```python
from build123d import *

# Parameters (mm, degrees)
SKETCH_1_W          = 120
SKETCH_1_H          = 40
EXTRUDE_1_DEPTH     = 25
SKETCH_2_R          = 2.75
CUT_EXTRUDE_1_DEPTH = 25
SKETCH_5_W          = 157.5
SKETCH_5_H          = 80
EXTRUDE_2_DEPTH     = 5
SKETCH_6_W          = 60
SKETCH_6_H          = 40
CUT_EXTRUDE_3_DEPTH = 20
FILLET_1_R          = 4
CHAMFER_1_SIZE      = 0.5


with BuildPart() as part:
    # 草图1 → 凸台-拉伸1 (new body)
    with BuildSketch(Plane(origin=(0, 0, 0), x_dir=(1, 0, 0), z_dir=(0, 1, 0))):
        Rectangle(SKETCH_1_W, SKETCH_1_H)
    extrude(amount=EXTRUDE_1_DEPTH)

    # 草图2 → 切除-拉伸1 (cut)
    with BuildSketch(Plane.XZ):
        with Locations(Location((-52.5, 11.75, 0), (0, 0, 270))):
            Circle(SKETCH_2_R)
        with Locations(Location((-52.5, -11.75, 0), (0, 0, 270))):
            Circle(SKETCH_2_R)
        with Locations(Location((52.5, -11.75, 0), (0, 0, 270))):
            Circle(SKETCH_2_R)
        with Locations(Location((52.5, 11.75, 0), (0, 0, 270))):
            Circle(SKETCH_2_R)
    extrude(amount=-CUT_EXTRUDE_1_DEPTH, mode=Mode.SUBTRACT)

    # 草图5 → 凸台-拉伸2 (add)
    with BuildSketch(Plane(origin=(0, 25, 0), x_dir=(1, 0, 0), z_dir=(0, 1, 0))):
        with Locations((0, 20)):
            Rectangle(SKETCH_5_W, SKETCH_5_H)
    extrude(amount=EXTRUDE_2_DEPTH)

    # 草图6 → 切除-拉伸3 (cut)
    with BuildSketch(Plane.XZ):
        Rectangle(SKETCH_6_W, SKETCH_6_H)
    extrude(amount=-CUT_EXTRUDE_3_DEPTH, mode=Mode.SUBTRACT)

    # 圆角1
    fillet_1_edges = [part.edges().sort_by_distance(p)[0] for p in [
        (-78.75, 27.5, -60),
        (-78.75, 27.5, 20),
        (78.75, 27.5, 20),
        (78.75, 27.5, -60),
    ]]
    fillet(fillet_1_edges, radius=FILLET_1_R)

    # 倒角1
    chamfer_1_edges = [part.edges().sort_by_distance(p)[0] for p in [
        (52.5, 0, 14.5),
        (52.5, 0, -9),
        (-52.5, 0, -9),
        (-52.5, 0, 14.5),
    ]]
    chamfer(chamfer_1_edges, length=CHAMFER_1_SIZE)


solid = part.part
```
Geometry check sheet. Reference: the model listing, model coordinates, mm. A direction names the side the tool comes from. Coordinates: 2 decimals unless noted, no trailing zeros. Order: outer loops, then holes, each group sorted by start corner. A loop starts at its lowest first (then second) coordinate and runs counter-clockwise, first axis right, second up. Notation, with made-up numbers: (12.5, 53) - (30.5, 53) arc R16 ccw to (30.5, 62) - close; hole circle Ø6 at (-33.5, 54.25). An arc over 180 degrees is marked (long way). Answer in a Markdown table with one row per item. Add a question column.
1. Material ranges on L1, parallel to X at y = 18.5, z = -11.75; L2, parallel to X at y = 6.5, z = -18; L3, parallel to Z at x = 59.5, y = 21.75, recorded low to high. Write a range as [from, to].
2. Section check B-B (x = -11). Enter the section's corners in (y, z).
3. Section check D-D (x = 52.5). Enter the section's corners in (y, z).
4. Draft check along Z on faces 4 (the face through (-77.609, 27.535, 18.797)), 5 (the face through (-53, 25, -12)), 6 (the face through (0, 20, 0)). Enter one of: +Z half, -Z half, draft (parallel to the pull), parting line (faces both ways), or undercut.
5. Section check A-A (y = 11.5). Enter the section's corners in (x, z), plus the area to 3 significant figures.
6. Access from +Z, -Z, +X, -X, +Y, -Y to the whole of each face (thin tool, end or side, straight path). Record for faces 1 (the face through (60, 12, 0)), 2 (the face through (-49.773, 12.578, -11.392)), 3 (the face through (-30, 10, 0)).
7. Gauge pin test, flat ends, axial feed: pin 1 Ø1.5 at (y, z) = (5, -2) entering from +X; pin 2 Ø2 at (y, z) = (14.5, -1.5) entering from -X; pin 3 Ø3.5 at (x, z) = (52.5, 11.75) entering from -Y. Record the tip position at first contact, or that the pin passes through.
8. Section check C-C (z = -11.75). Enter the section's corners in (x, y).
Data:
| question | item | result |
|---|---|---|
| 1 | L1 | x = [-60, -55.25], [-49.75, -30], [30, 49.75], [55.25, 60] |
| 1 | L2 | x = [-60, -30], [30, 60] |
| 1 | L3 | z = [-20, 20] |
| 2 | outline | (20, -20) - (25, -20) - (25, -60) - (30, -60) - (30, 20) - (20, 20) - close |
| 3 | outline | (0, -20) - (25, -20) - (25, -60) - (30, -60) - (30, 20) - (0, 20) - (0, 15) - (0.5, 14.5) - (25, 14.5) - (25, 9) - (0.5, 9) - (0, 8.5) - (0, -8.5) - (0.5, -9) - (25, -9) - (25, -14.5) - (0.5, -14.5) - (0, -15) - close |
| 4 | face 4 | +Z half |
| 4 | face 5 | undercut |
| 4 | face 6 | draft |
| 5 | outline | (-60, -20) - (-30, -20) - (-30, 20) - (-60, 20) - close; (30, -20) - (60, -20) - (60, 20) - (30, 20) - close; hole circle Ø5.5 at (-52.5, -11.75); hole circle Ø5.5 at (-52.5, 11.75); hole circle Ø5.5 at (52.5, -11.75); hole circle Ø5.5 at (52.5, 11.75) |
| 5 | area | 2,300 mm² |
| 6 | face 1 | +Z, -Z, +X, -Y |
| 6 | face 2 | -Y |
| 6 | face 3 | +Z, -Z, -Y |
| 7 | pin 1 | stops at x = 60 |
| 7 | pin 2 | stops at x = -60 |
| 7 | pin 3 | stops at y = 25 |
| 8 | outline | (-78.75, 25) - (-60, 25) - (-60, 0) - (-55.75, 0) - (-55.25, 0.5) - (-55.25, 25) - (-49.75, 25) - (-49.75, 0.5) - (-49.25, 0) - (-30, 0) - (-30, 20) - (30, 20) - (30, 0) - (49.25, 0) - (49.75, 0.5) - (49.75, 25) - (55.25, 25) - (55.25, 0.5) - (55.75, 0) - (60, 0) - (60, 25) - (78.75, 25) - (78.75, 30) - (-78.75, 30) - close |
